```python
from build123d import *

# Parameters (mm, degrees)
BOSS_EXTRUDE1_DEPTH       = 3.175
FILLET1_R                 = 25.4
FILLET2_R                 = 3.175
FILLET3_R                 = 3.175
F_2_56_TAPPED_HOLE1_D     = 1.778
F_2_56_TAPPED_HOLE1_DEPTH = 5.588
F_2_56_TAPPED_HOLE1_TIP   = 0.53416509
F_2_CLEARANCE_HOLE1_D     = 2.4384
F_2_CLEARANCE_HOLE1_DEPTH = 25.4
F_2_CLEARANCE_HOLE1_TIP   = 0.732569267
SKETCH12_W                = 1.5875
SKETCH12_H                = 3.175
CUT_EXTRUDE1_DEPTH        = 3.175
F_2_56_TAPPED_HOLE2_D     = 1.778
F_2_56_TAPPED_HOLE2_DEPTH = 5.588
F_2_56_TAPPED_HOLE2_TIP   = 0.53416509
F_2_56_TAPPED_HOLE3_D     = 1.778
F_2_56_TAPPED_HOLE3_DEPTH = 5.588
F_2_56_TAPPED_HOLE3_TIP   = 0.53416509
F_2_56_TAPPED_HOLE4_D     = 1.778
F_2_56_TAPPED_HOLE4_DEPTH = 10.668
F_2_56_TAPPED_HOLE4_TIP   = 0.53416509


with BuildPart() as part:
    # Sketch1 → Boss-Extrude1 (new body, symmetric)
    with BuildSketch(Plane.XY):
        Polygon((0, 38.1), (0, 0), (63.5, 0), (63.5, 65.659), (25.4, 65.659), align=None)
    extrude(amount=BOSS_EXTRUDE1_DEPTH, both=True)

    # Fillet1
    fillet1_edges = [part.edges().sort_by_distance(p)[0] for p in [
        (25.4, 65.659, 0),
    ]]
    fillet(fillet1_edges, radius=FILLET1_R)

    # Fillet2
    fillet2_edges = [part.edges().sort_by_distance(p)[0] for p in [
        (0, 38.1, 0),
    ]]
    fillet(fillet2_edges, radius=FILLET2_R)

    # Fillet3
    fillet3_edges = [part.edges().sort_by_distance(p)[0] for p in [
        (63.5, 65.659, 0),
    ]]
    fillet(fillet3_edges, radius=FILLET3_R)

    # #2-56 Tapped Hole1
    with Locations(Plane(origin=(63.5, 0, 0), x_dir=(0, 0, -1), z_dir=(1, 0, 0))):
        with Locations((0, 50.796059009), (0, 19.476973799)):
            Hole(F_2_56_TAPPED_HOLE1_D / 2, depth=F_2_56_TAPPED_HOLE1_DEPTH)
            with Locations((0, 0, -(F_2_56_TAPPED_HOLE1_DEPTH + F_2_56_TAPPED_HOLE1_TIP / 2))):  # 118° drill point
                Cone(0, F_2_56_TAPPED_HOLE1_D / 2, F_2_56_TAPPED_HOLE1_TIP, mode=Mode.SUBTRACT)

    # #2 Clearance Hole1
    with Locations(Plane.XY.offset(3.175)):
        with Locations((57.15, 40.259), (44.45, 40.259)):
            Hole(F_2_CLEARANCE_HOLE1_D / 2, depth=F_2_CLEARANCE_HOLE1_DEPTH)
            with Locations((0, 0, -(F_2_CLEARANCE_HOLE1_DEPTH + F_2_CLEARANCE_HOLE1_TIP / 2))):  # 118° drill point
                Cone(0, F_2_CLEARANCE_HOLE1_D / 2, F_2_CLEARANCE_HOLE1_TIP, mode=Mode.SUBTRACT)

    # Sketch12 → Cut-Extrude1 (cut)
    with BuildSketch(Plane(origin=(0, 0, -3.175), x_dir=(-1, 0, 0), z_dir=(0, 0, -1))):
        with Locations((-2.38125, 23.8125)):
            Rectangle(SKETCH12_W, SKETCH12_H)
        with Locations((-2.38125, 11.1125)):
            Rectangle(SKETCH12_W, SKETCH12_H)
    extrude(amount=-CUT_EXTRUDE1_DEPTH, mode=Mode.SUBTRACT)

    # #2-56 Tapped Hole2
    with Locations(Plane(origin=(-18.986783635, 17.499339756, 0), x_dir=(0, 0, 1), z_dir=(-0.735322884, 0.677716944, 0))):
        with Locations((0, 41.828773603)):
            Hole(F_2_56_TAPPED_HOLE2_D / 2, depth=F_2_56_TAPPED_HOLE2_DEPTH)
            with Locations((0, 0, -(F_2_56_TAPPED_HOLE2_DEPTH + F_2_56_TAPPED_HOLE2_TIP / 2))):  # 118° drill point
                Cone(0, F_2_56_TAPPED_HOLE2_D / 2, F_2_56_TAPPED_HOLE2_TIP, mode=Mode.SUBTRACT)

    # #2-56 Tapped Hole3
    with Locations(Plane(origin=(0, 65.659, 0), x_dir=(-1, 0, 0), z_dir=(0, 1, 0))):
        with Locations((-48.407010359, 0)):
            Hole(F_2_56_TAPPED_HOLE3_D / 2, depth=F_2_56_TAPPED_HOLE3_DEPTH)
            with Locations((0, 0, -(F_2_56_TAPPED_HOLE3_DEPTH + F_2_56_TAPPED_HOLE3_TIP / 2))):  # 118° drill point
                Cone(0, F_2_56_TAPPED_HOLE3_D / 2, F_2_56_TAPPED_HOLE3_TIP, mode=Mode.SUBTRACT)

    # #2-56 Tapped Hole4
    with Locations(Plane.XY.offset(3.175)):
        with Locations((3.175, 33.3375)):
            Hole(F_2_56_TAPPED_HOLE4_D / 2, depth=F_2_56_TAPPED_HOLE4_DEPTH)
            with Locations((0, 0, -(F_2_56_TAPPED_HOLE4_DEPTH + F_2_56_TAPPED_HOLE4_TIP / 2))):  # 118° drill point
                Cone(0, F_2_56_TAPPED_HOLE4_D / 2, F_2_56_TAPPED_HOLE4_TIP, mode=Mode.SUBTRACT)


solid = part.part
```
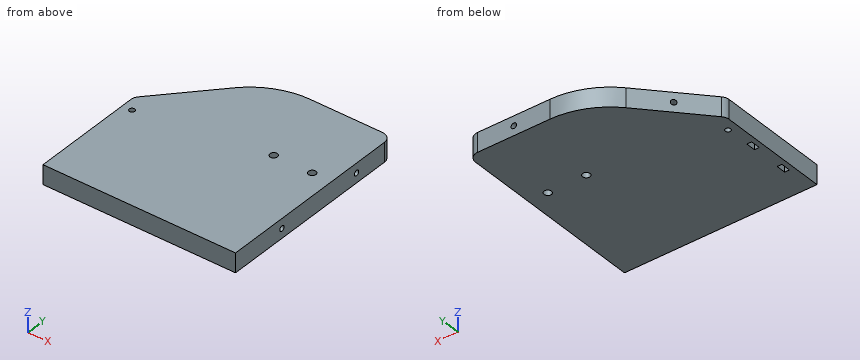
The listing builds one solid part. Answer for the finished solid, in the listing's coordinates (mm). Give positions to 0.01 mm unless a question says otherwise; leave off trailing zeros. Order: outer loops, then holes, each group sorted by start corner. A loop starts at its lowest first (then second) coordinate and runs counter-clockwise, first axis right, second up. Notation, with made-up numbers: (87.5, 54) -> (136.5, 54) arc R3 ccw to (136.5, 58) -> close; hole circle Ø8 at (13, -18.5). An arc over 180 degrees is marked (long way). Answer as a JSON object with one key per item and string values. Group by question number.
Item 1: The part is cut by section A-A on x = 44.45. Write down the section's boundary in (y, z) (3 decimals).
Item 2: The part is cut by section B-B on y = 52.5. Write down the section's boundary in (x, z) (3 decimals).
Item 3: Consider L1, parallel to Y at x = 59.6, z = 0; L2, parallel to X at y = 40, z = 1.75; L3, parallel to Y at x = 3.5, z = 0. Determine where each line is inside the solid, lowest interval first. Write a range as from..to.
Item 4: Flat-ended cylindrical pins translate along their axes: pin 1 (1.3 mm diameter, centred on x = 2.5, z = -1.5, fed in from +Y); pin 2 (2 mm diameter, centred on x = 44.45, y = 40.259, fed in from -Z). Find the tip coordinate at first contact, or state that the pin passes through.
Result set:
{
 "1": {"outline": "(0, -3.175) -> (39.04, -3.175) -> (39.04, 3.175) -> (0, 3.175) -> close; (41.478, -3.175) -> (65.659, -3.175) -> (65.659, 3.175) -> (41.478, 3.175) -> close"},
 "2": {"outline": "(13.272, -3.175) -> (63.5, -3.175) -> (63.5, 3.175) -> (13.272, 3.175) -> close"},
 "3": {"L1": "0..18.59, 20.37..49.91, 51.69..65.66", "L2": "1.75..43.26, 45.64..55.96, 58.34..63.5", "L3": "0..32.51, 34.16..41.9"},
 "4": {"pin 1": "y = 41.52", "pin 2": "through"}
}
